The model under review builds one solid part; all positions refer to its coordinate system, in mm. Face numbers are marked on the shaded views. A direction names the side the tool comes from. Give positions to 0.01 mm unless a question says otherwise; leave off trailing zeros. Return JSON: item names as keys, results as strings. Group by question number.
```python
from build123d import *

# Parameters (mm, degrees)
SKETCH_1_R          = 4.2
EXTRUDE_1_DEPTH     = 2.9
SKETCH_2_R          = 2.5
EXTRUDE_2_DEPTH     = 8
CUT_EXTRUDE_1_DEPTH = 6.4


with BuildPart() as part:
    # 草图1 → 凸台-拉伸1 (new body)
    with BuildSketch(Plane(origin=(0, 0, 0), x_dir=(1, 0, 0), z_dir=(0, 1, 0))):
        Circle(SKETCH_1_R)
    extrude(amount=EXTRUDE_1_DEPTH)

    # 草图2 → 凸台-拉伸2 (add)
    with BuildSketch(Plane(origin=(0, 2.9, 0), x_dir=(1, 0, 0), z_dir=(0, 1, 0))):
        Circle(SKETCH_2_R)
    extrude(amount=EXTRUDE_2_DEPTH)

    # 草图3 one side → 切除-旋转1 (revolve, cut)
    with BuildSketch(Plane(origin=(0, 0, 0), x_dir=(0, 0, -1), z_dir=(1, 0, 0))):
        with BuildLine():
            ThreePointArc((0, 0), (-2.24147848, 0.330353936), (-4.2, 1.469455754))
            Line((-4.2, 1.469455754), (-5.100943616, -0.95254451))
            Line((-5.100943616, -0.95254451), (0, -0.95254451))
            Line((0, -0.95254451), (0, 0))
        make_face()
    revolve(axis=Axis((0, 1.035939113, 0), (0, -1, 0)), mode=Mode.SUBTRACT)

    # 草图4 → 切除-拉伸1 (cut)
    with BuildSketch(Plane(origin=(0, -5, 0), x_dir=(1, 0, 0), z_dir=(0, 1, 0))):
        Polygon((0.4, -2.5), (0.4, -0.4), (2.5, -0.4), (2.5, 0.4), (0.4, 0.4), (0.4, 2.5), (-0.4, 2.5), (-0.4, 0.4), (-2.5, 0.4), (-2.5, -0.4), (-0.4, -0.4), (-0.4, -2.5), align=None)
    extrude(amount=CUT_EXTRUDE_1_DEPTH, mode=Mode.SUBTRACT)


solid = part.part
```
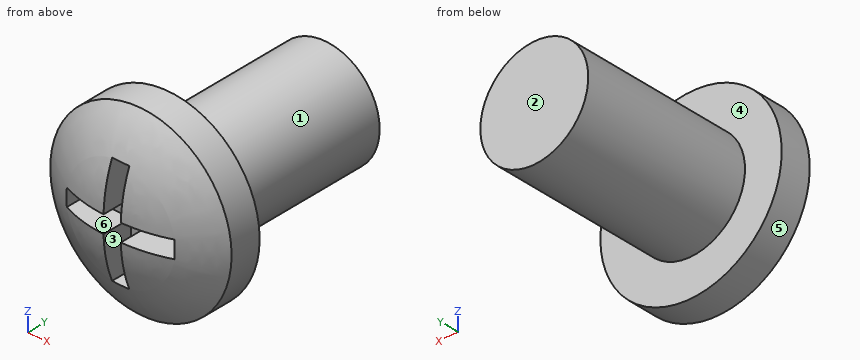
(1) For probe 1 along Z at (x, y) = (0, 7.75); probe 2 along Y at (x, z) = (-1.75, 1.25); probe 3 along Y at (x, z) = (2.5, 3.25), list the stretches that pass through material, from the lowest coordinate up.
(2) For pin 1 (1 mm diameter, centred on y = 3.5, z = 2, fed in from -X); pin 2 (1 mm diameter, centred on x = 3.5, y = 2.5, fed in from -Z); pin 3 (1.5 mm diameter, centred on x = -1.5, y = 0.5, fed in from +Z), all flat-tipped, find the tip position at first contact; note any pin that passes through.
(3) Mouldability with a two-part tool opening along Z and no side actions: class the marked faces 4, 5 and 6 as released by +Z, released by -Z, zero draft, split by the parting line, or undercut.
(4) For the marked faces 1, 2 and 3, list the 3-axis set-ups (+Z, -Z, +X, -X, +Y, -Y) from which the entire face can be reached by the end or side of a thin tool; tool diameter is ignored.
Verdict:
{
 "1": {"probe 1": "z = -2.5 to 2.5", "probe 2": "y = 0.3 to 10.9", "probe 3": "y = 1.38 to 2.9"},
 "2": {"pin 1": "stops at x = -2", "pin 2": "stops at z = -2.94", "pin 3": "stops at z = 3.67"},
 "3": {"face 4": "zero draft", "face 5": "split by the parting line", "face 6": "undercut"},
 "4": {"face 1": "+Y", "face 2": "+Z, -Z, +X, -X, +Y", "face 3": "-Y"}
}
